Source: CAD feature listing. Evaluate the final solid. Frame: model axes, mm. Round coordinates to 2 decimals unless told otherwise and drop trailing zeros. Loops run counter-clockwise (first coordinate to the right, second up) from the corner with the lowest first, then second, coordinate; pieces in that order, holes last.
(1) Section A-A, the plane z = 5.25. Return the cut outline in (x, y).
(2) First-contact query: pin 1 Ø6 at (x, z) = (-8, 13.5) entering from -Y; pin 2 Ø4 at (x, z) = (22.5, 7) entering from +Y; pin 3 Ø1.5 at (x, z) = (-32.5, 5) entering from -Y. Flat tips, straight axial feed; report the tip coordinate or a pass-through.
(3) Material intervals for probe 1 along Y at (x, z) = (0, 9.75); probe 2 along X at (y, z) = (-7, 9.75); probe 3 along X at (y, z) = (-8.5, 12.25), sorted ascending.
```python
from build123d import *

# Parameters (mm, degrees)
SKETCH1_R      = 47.5
SKETCH1_R_2    = 30
EXTRUDE1_DEPTH = 18
CHAMFER1_SIZE  = 1


with BuildPart() as part:
    # Sketch1 → Extrude1 (new body)
    with BuildSketch(Plane.XY):
        Circle(SKETCH1_R)
        Circle(SKETCH1_R_2, mode=Mode.SUBTRACT)
    extrude(amount=EXTRUDE1_DEPTH)

    # Chamfer1
    chamfer1_edges = [part.edges().sort_by_distance(p)[0] for p in [
        (-47.5, 0, 0),
        (-47.5, 0, 18),
        (-30, 0, 0),
        (-30, 0, 18),
    ]]
    chamfer(chamfer1_edges, length=CHAMFER1_SIZE)

    # Sketch2 → Cut-Revolve1 (revolve, cut)
    with BuildSketch(Plane(origin=(0, 0, 0), x_dir=(0, 0, -1), z_dir=(1, 0, 0))):
        Polygon((-18, 35.5), (-17.65, 35.85), (-18, 36.2), align=None)
        Polygon((-17.65, 44.35), (-18, 44), (-18, 44.7), align=None)
        Polygon((0, 35.5), (0, 36.2), (-0.35, 35.85), align=None)
        Polygon((0, 44.7), (0, 44), (-0.35, 44.35), align=None)
    revolve(axis=Axis((0, 0, 0), (0, 0, 1)), mode=Mode.SUBTRACT)


solid = part.part
```
Output values:
1. outline: circle Ø95 at (0, 0); hole circle Ø60 at (0, 0)
2. pin 1: stops at y = -47.24
2. pin 2: stops at y = 42.85
2. pin 3: stops at y = -35.33
3. probe 1: y = -47.5 to -30, 30 to 47.5
3. probe 2: x = -46.98 to -29.17, 29.17 to 46.98
3. probe 3: x = -46.73 to -28.77, 28.77 to 46.73
